```python
from build123d import *

# Parameters (mm, degrees)
F0_R      = 5.715
F0_R_2    = 4.445
F1_DEPTH  = 52.8
F2_R      = 24.13
F2_R_2    = 5.715
F3_DEPTH  = 2.54
F4_R      = 24.13
F4_R_2    = 5.715
F5_DEPTH  = 2.54
F6_R      = 1.25
F7_DEPTH  = 52.801
F8_R      = 18.13
F8_R_2    = 4.445
F9_DEPTH  = 2.54
F10_R     = 1.5
F11_R     = 4.445
F12_DEPTH = 2.54
F13_R     = 18.13
F13_R_2   = 4.445
F14_DEPTH = 2.54
F15_R     = 1.5
F16_R     = 4.445
F17_DEPTH = 2.54
F18_R     = 1.25
F19_DEPTH = 57.881


with BuildPart() as f1:
    # F0 (on Top) → F1 (new body)
    with BuildSketch(Plane.XY):
        Circle(F0_R)
        Circle(F0_R_2, mode=Mode.SUBTRACT)
    extrude(amount=F1_DEPTH)

    # F2 (on face) → F3 (join)
    with BuildSketch(Plane.XY.offset(52.8)):
        Circle(F2_R)
        Circle(F2_R_2, mode=Mode.SUBTRACT)
    extrude(amount=-F3_DEPTH)

    # F4 (on face) → F5 (join)
    with BuildSketch(Plane(origin=(0, 0, 0), x_dir=(1, 0, 0), z_dir=(0, 0, -1))):
        Circle(F4_R)
        Circle(F4_R_2, mode=Mode.SUBTRACT)
    extrude(amount=-F5_DEPTH)

    # F6 (on face) → F7 (cut, through all)
    with BuildSketch(Plane(origin=(0, 0, 0), x_dir=(1, 0, 0), z_dir=(0, 0, -1))):
        with Locations((-21.13, 0)):
            Circle(F6_R)
        with Locations((-14.941166, -14.941166)):
            Circle(F6_R)
        with Locations((0, -21.13)):
            Circle(F6_R)
        with Locations((14.941166, -14.941166)):
            Circle(F6_R)
        with Locations((21.13, 0)):
            Circle(F6_R)
        with Locations((14.941166, 14.941166)):
            Circle(F6_R)
        with Locations((0, 21.13)):
            Circle(F6_R)
        with Locations((-14.941166, 14.941166)):
            Circle(F6_R)
    extrude(amount=-F7_DEPTH, mode=Mode.SUBTRACT)

    # F8 (on face) → F9 (join)
    with BuildSketch(Plane(origin=(0, 0, 0), x_dir=(1, 0, 0), z_dir=(0, 0, -1))):
        Circle(F8_R)
        Circle(F8_R_2, mode=Mode.SUBTRACT)
    extrude(amount=F9_DEPTH)

    # F10
    f10_edges = [f1.edges().sort_by_distance(p)[0] for p in [
        (-18.13, 0, -2.54),
    ]]
    fillet(f10_edges, radius=F10_R)

    # F11 (on face) → F12 (cut)
    with BuildSketch(Plane(origin=(0, 0, -2.54), x_dir=(1, 0, 0), z_dir=(0, 0, -1))):
        Polygon((3.727945, 9.000055), (0, 12.728), (-3.727945, 9.000055), (-9.000055, 9.000055), (-9.000055, 3.727945), (-12.728, 0), (-9.000055, -3.727945), (-9.000055, -9.000055), (-3.727945, -9.000055), (0, -12.728), (3.727945, -9.000055), (9.000055, -9.000055), (9.000055, -3.727945), (12.728, 0), (9.000055, 3.727945), (9.000055, 9.000055), align=None)
        Circle(F11_R, mode=Mode.SUBTRACT)
        Circle(F11_R)
    extrude(amount=-F12_DEPTH, mode=Mode.SUBTRACT)

    # F13 (on face) → F14 (join)
    with BuildSketch(Plane.XY.offset(52.8)):
        Circle(F13_R)
        Circle(F13_R_2, mode=Mode.SUBTRACT)
    extrude(amount=F14_DEPTH)

    # F15
    f15_edges = [f1.edges().sort_by_distance(p)[0] for p in [
        (-18.13, 0, 55.34),
    ]]
    fillet(f15_edges, radius=F15_R)

    # F16 (on face) → F17 (cut)
    with BuildSketch(Plane.XY.offset(55.34)):
        Polygon((3.727945, 9.000055), (0, 12.728), (-3.727945, 9.000055), (-9.000055, 9.000055), (-9.000055, 3.727945), (-12.728, 0), (-9.000055, -3.727945), (-9.000055, -9.000055), (-3.727945, -9.000055), (0, -12.728), (3.727945, -9.000055), (9.000055, -9.000055), (9.000055, -3.727945), (12.728, 0), (9.000055, 3.727945), (9.000055, 9.000055), align=None)
        Circle(F16_R, mode=Mode.SUBTRACT)
    extrude(amount=-F17_DEPTH, mode=Mode.SUBTRACT)

    # F18 (on face) → F19 (cut, through all)
    with BuildSketch(Plane.XY.offset(55.34)):
        with Locations((-12.141246, 5.029069)):
            Circle(F18_R)
        with Locations((-12.141246, -5.029069)):
            Circle(F18_R)
        with Locations((-5.029069, -12.141246)):
            Circle(F18_R)
        with Locations((5.029069, -12.141246)):
            Circle(F18_R)
        with Locations((12.141246, -5.029069)):
            Circle(F18_R)
        with Locations((12.141246, 5.029069)):
            Circle(F18_R)
        with Locations((5.029069, 12.141246)):
            Circle(F18_R)
        with Locations((-5.029069, 12.141246)):
            Circle(F18_R)
    extrude(amount=-F19_DEPTH, mode=Mode.SUBTRACT)


solid = f1.part
```
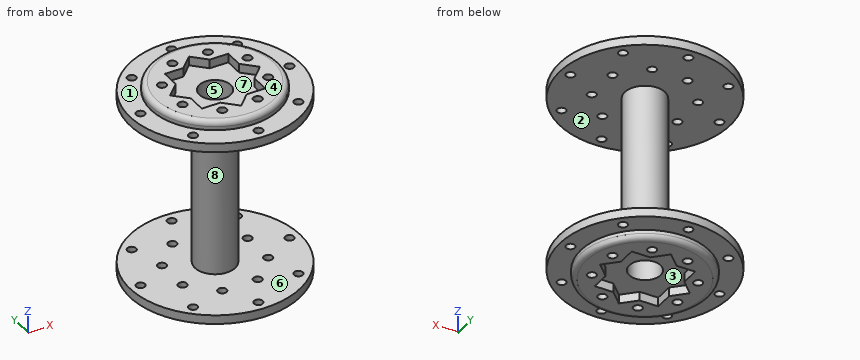
Read the model definition and answer for the solid it produces. Units are mm, in the model's axes. Face numbers are marked on the shaded views. A direction names the side the tool comes from. Coordinates: 2 decimals unless noted, no trailing zeros. Write each loop counter-clockwise with the first axis right and the second up, starting at its lowest first coordinate (ties: lowest second). Pieces come first, ordered by that corner, then holes. Notation, with made-up numbers: (87, 31) - (114, 31) arc R22 ccw to (114, 56) - close; hole circle Ø5 at (2.5, 71). An arc over 180 degrees is marked (long way). Answer as a JSON object with one key per item and string values. Group by question number.
1. Each of these flat-tipped pins is pushed along its axis until it touches: P1, Ø1.5, axis at x = 14.94, y = 14.94, coming from the +Z side; P2, Ø1.3, axis at y = 6, z = 54.5, coming from the -X side; P3, Ø6, axis at x = 13.5, y = -17, coming from the +Z side; P4, Ø4, axis at x = 0, y = -21.13, coming from the -Z side. Where does it stop, or does it pass through?
2. Consider L1, parallel to Y at x = 0, z = 2.05 (3 decimals); L2, parallel to Z at x = -3, y = 6; L3, parallel to Z at x = 1.5, y = -14. Determine where each line is inside the solid, lowest interval first. Write a range as [from, to].
3. A cutting plane is placed at B-B (z = 12). Determine the outline of the cut face in (x, y) (3 decimals).
4. A cutting plane is placed at D-D (z = 1). Give the number of separate pieces and of enclosed holes in the cut face, plus the area to 3 significant figures.
5. Which of the six approach directions +Z, -Z, +X, -X, +Y, -Y give full straight-line access (tool end or side, diameter ignored) to the marked faces 1, 2, 3 and 4?
6. A cutting plane is placed at A-A (y = -21.13). Determine the outline of the cut face in (x, z).
7. The mould has two halves that part along Y. Classify the marked faces 5, 6, 7 and 8: +Y half, -Y half, draft (parallel to the pull), parting line (faces both ways), or undercut.
Worked out:
{
 "1": {"P1": "passes through", "P2": "stops at x = -17.26", "P3": "stops at z = 52.8", "P4": "stops at z = 0"},
 "2": {"L1": "y = [-24.13, -22.38], [-19.88, -4.445], [4.445, 19.88], [22.38, 24.13]", "L2": "z = [0, 2.54], [50.26, 52.8]", "L3": "z = [-2.54, 2.54], [50.26, 55.34]"},
 "3": {"outline": "circle Ø11.43 at (0, 0); hole circle Ø8.89 at (0, 0)"},
 "4": {"separate pieces": "1", "enclosed holes": "17", "area": "1,690 mm²"},
 "5": {"face 1": "+Z", "face 2": "none", "face 3": "-Z", "face 4": "+Z, +X, -X, +Y, -Y"},
 "6": {"outline": "(-11.65, 0) - (-1.25, 0) - (-1.25, 2.54) - (-11.65, 2.54) - close; (-11.65, 50.26) - (-1.25, 50.26) - (-1.25, 52.8) - (-11.65, 52.8) - close; (1.25, 0) - (11.65, 0) - (11.65, 2.54) - (1.25, 2.54) - close; (1.25, 50.26) - (11.65, 50.26) - (11.65, 52.8) - (1.25, 52.8) - close"},
 "7": {"face 5": "undercut", "face 6": "draft", "face 7": "undercut", "face 8": "parting line"}
}
